Part print with two shaded views. Sizes in mm from the minimum x, y, z corner. A direction names the side the tool comes from. Coordinates: 2 decimals unless noted, no trailing zeros. Loops run counter-clockwise (first coordinate to the right, second up) from the corner with the lowest first, then second, coordinate; pieces in that order, holes last. Notation, with made-up numbers: (-19.5, -19.75) - (26.5, -19.75) arc R35 cw to (26.5, 18.25) - close; hole circle Ø7 at (80, -24.5). An arc over 180 degrees is marked (long way). Answer as CSV lines item,"result".
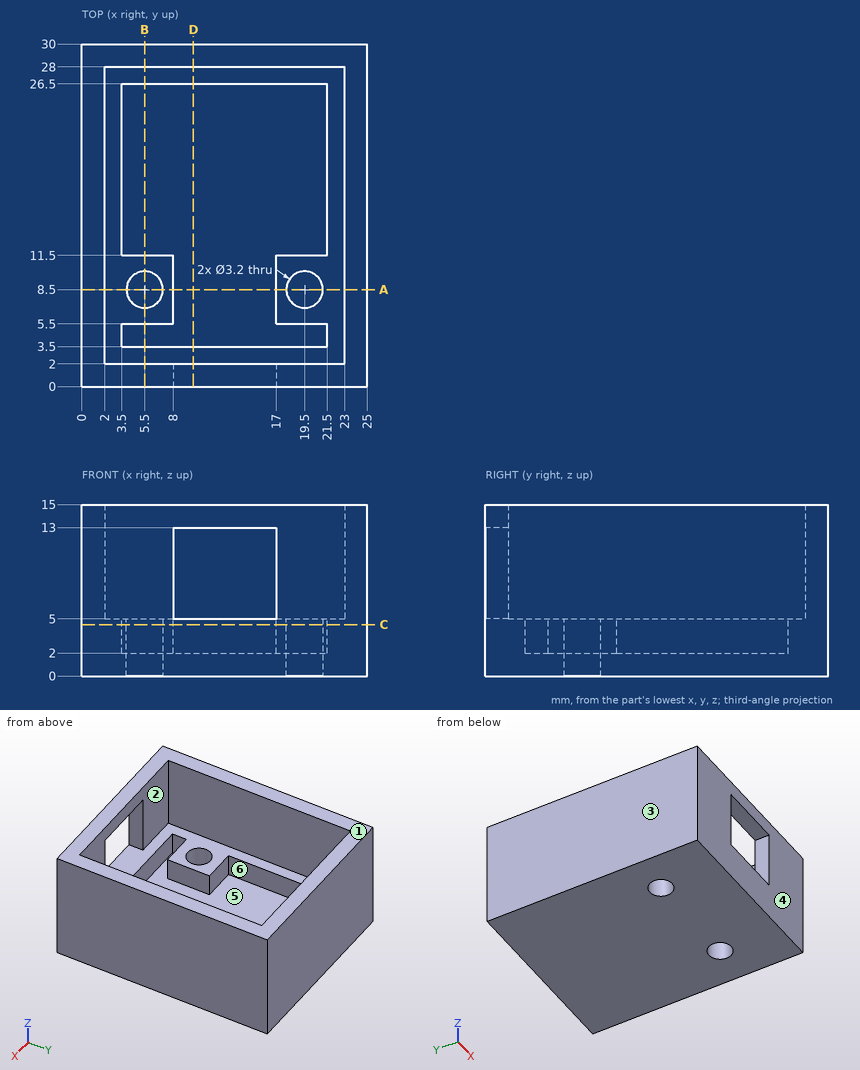
Q1. Saw through at D-D (x = 9.75). Give the cut face in (y, z).
Results:
outline,"(0, 0) - (30, 0) - (30, 15) - (28, 15) - (28, 5) - (26.5, 5) - (26.5, 2) - (3.5, 2) - (3.5, 5) - (0, 5) - close; (0, 13) - (2, 13) - (2, 15) - (0, 15) - close"
Q2. Saw through at C-C (z = 4.5). Give the cut face in (x, y), then the cut area to 3 significant figures.
Results:
outline,"(0, 0) - (25, 0) - (25, 30) - (0, 30) - close; hole (3.5, 3.5) - (21.5, 3.5) - (21.5, 5.5) - (17, 5.5) - (17, 11.5) - (21.5, 11.5) - (21.5, 26.5) - (3.5, 26.5) - (3.5, 11.5) - (8, 11.5) - (8, 5.5) - (3.5, 5.5) - close; hole circle Ø3.2 at (5.5, 8.5); hole circle Ø3.2 at (19.5, 8.5)"
area,"374 mm^2"
Q3. Wall check: L1, parallel to Y at x = 19.5, z = 3.15; L2, parallel to X at y = 3, z = 9.75; L3, parallel to X at y = 17.25, z = 3.25. Give the ranges that are in metal, low to high.
Results:
L1,"y = 0 to 3.5, 5.5 to 6.9, 10.1 to 11.5, 26.5 to 30"
L2,"x = 0 to 2, 23 to 25"
L3,"x = 0 to 3.5, 21.5 to 25"
Q4. Saw through at A-A (y = 8.5). Give the cut face in (x, z), then the cut area to 3 significant figures.
Results:
outline,"(0, 0) - (3.9, 0) - (3.9, 5) - (2, 5) - (2, 15) - (0, 15) - close; (7.1, 0) - (17.9, 0) - (17.9, 5) - (17, 5) - (17, 2) - (8, 2) - (8, 5) - (7.1, 5) - close; (21.1, 0) - (25, 0) - (25, 15) - (23, 15) - (23, 5) - (21.1, 5) - close"
area,"106 mm^2"
Q5. Two-plate mould, pull along X, no slides. Class the marked faces 3, 4, 5 and 6: released by +X, released by -X, zero draft, split by the parting line, or undercut.
Results:
face 3,"released by -X"
face 4,"zero draft"
face 5,"undercut"
face 6,"undercut"
Q6. Which spindle directions (+Z, -Z, +X, -X, +Y, -Y) get a long thin tool onto all of the face, cutting with end or side? Do the marked faces 1 and 2. Say none if no direction does.
Results:
face 1,"+Z, +X, -X, +Y, -Y"
face 2,"+Z"
Q7. Saw through at B-B (x = 5.5). Give the cut face in (y, z).
Results:
outline,"(0, 0) - (6.9, 0) - (6.9, 5) - (5.5, 5) - (5.5, 2) - (3.5, 2) - (3.5, 5) - (2, 5) - (2, 15) - (0, 15) - close; (10.1, 0) - (30, 0) - (30, 15) - (28, 15) - (28, 5) - (26.5, 5) - (26.5, 2) - (11.5, 2) - (11.5, 5) - (10.1, 5) - close"
Q8. Flat gauge pins, fed straight in: pin 1 (14.5 mm diameter, centred on x = 14, y = 20.5, fed in from +Z); pin 2 (3 mm diameter, centred on x = 10, y = 19.5, fed in from +Z). Where does each tip first touch, or does it go through?
Results:
pin 1,"stops at z = 5"
pin 2,"stops at z = 2"
